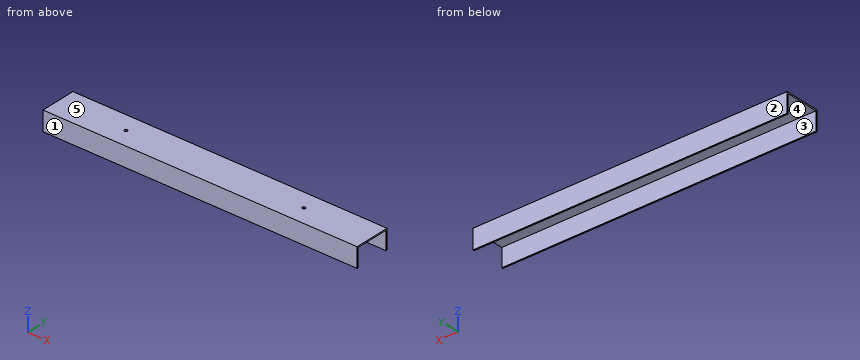
from build123d import *

# Parameters (mm, degrees)
F0_W     = 615.95
F0_H     = 69.85
F1_DEPTH = 19.05
F2_T     = -2.54
F3_R     = 3.175
F4_DEPTH = 38.101


with BuildPart() as f1:
    # F0 (on Top) → F1 (new body, symmetric)
    with BuildSketch(Plane.XY):
        Rectangle(F0_W, F0_H)
    extrude(amount=F1_DEPTH, both=True)

    # F2
    f2_openings = [f1.faces().sort_by_distance(p)[0] for p in [
        (0, 0, -19.05),
        (307.975, 0, 0),
        (-307.975, 0, 0),
    ]]
    offset(amount=F2_T, openings=f2_openings)

    # F3 (on face) → F4 (cut, through all)
    with BuildSketch(Plane.XY.offset(19.05)):
        with Locations((-174.244, 0)):
            Circle(F3_R)
        with Locations((174.244, 0)):
            Circle(F3_R)
    extrude(amount=-F4_DEPTH, mode=Mode.SUBTRACT)


solid = f1.part
Verification items for the finished model (mm, model axes). Face numbers are marked on the shaded views. A direction names the side the tool comes from. Coordinates: 2 decimals unless noted, no trailing zeros. Write each loop counter-clockwise with the first axis right and the second up, starting at its lowest first coordinate (ties: lowest second). Pieces come first, ordered by that corner, then holes. Notation, with made-up numbers: M 5,60.5 L 45,60.5 A28 ccw 45,82.5 Z; hole C -39.5,-11 d11. An arc over 180 degrees is marked long. One line per question, with ' | ' between items.
1) Release check for a two-part mould opening along Y. For the marked faces 1, 2 and 3 record: +Y half, -Y half, draft (parallel to the pull), parting line (faces both ways), or undercut.
Solutions:
face 1: -Y half | face 2: +Y half | face 3: undercut
2) Sectioned sample at A-A on z = -10.5. Record the cut outline in (x, y) (3 decimals).
Solutions:
outline: M -307.975,-34.925 L 307.975,-34.925 L 307.975,-32.385 L -307.975,-32.385 Z; M -307.975,32.385 L 307.975,32.385 L 307.975,34.925 L -307.975,34.925 Z
3) Access from +Z, -Z, +X, -X, +Y, -Y to the whole of each face (thin tool, end or side, straight path). Record for the marked faces 4 and 5.
Solutions:
face 4: -Z, +X, -X | face 5: +Z, +X, -X, +Y, -Y
4) Material ranges on L1, parallel to Y at x = 147, z = 4.5 (3 decimals); L2, parallel to Z at x = -249, y = 22, recorded low to high.
Solutions:
L1: -34.925 to -32.385, 32.385 to 34.925 | L2: 16.51 to 19.05
5) Sectioned sample at B-B on x = 29. Record the cut outline in (y, z) (3 decimals), then the cut area to 3 significant figures.
Solutions:
outline: M -34.925,-19.05 L -32.385,-19.05 L -32.385,16.51 L 32.385,16.51 L 32.385,-19.05 L 34.925,-19.05 L 34.925,19.05 L -34.925,19.05 Z | area: 358 mm^2
6) Sectioned sample at C-C on y = 24. Record the cut outline in (x, z) (3 decimals), then the cut area to 3 significant figures.
Solutions:
outline: M -307.975,16.51 L 307.975,16.51 L 307.975,19.05 L -307.975,19.05 Z | area: 1,560 mm^2
7) Depth check by flat-ended pin: pin 1 Ø1.5 at (x, y) = (-2, 6) entering from -Z. Enter the tip coordinate at first touch or a pass-through.
Solutions:
pin 1: z = 16.51
